The model under review builds one solid part; all positions refer to its coordinate system, in mm. A direction names the side the tool comes from. Round coordinates to 2 decimals unless told otherwise and drop trailing zeros. Loops run counter-clockwise (first coordinate to the right, second up) from the corner with the lowest first, then second, coordinate; pieces in that order, holes last. Notation, with made-up numbers: (88.5, 84) -> (130.5, 84) arc R22 ccw to (130.5, 92) -> close; hole circle Ø10 at (19, 9.5). An arc over 180 degrees is marked (long way). Use a Markdown table: item, result. Add a question column.
1) Wall thickness on probe 1 along Z at (x, y) = (-42.5, -19.5); probe 2 along Z at (x, y) = (1.5, -31.5); probe 3 along Z at (x, y) = (-49.5, -9): over which ranges is each line inside the solid? List them lowest first.
2) For faces 1 (the cylindrical face through (74.51, -17.26, -110.81)), 2 (the flat face through (-23, -25, 85)), list the 3-axis set-ups (+Z, -Z, +X, -X, +Y, -Y) from which the entire face can be reached by the end or side of a thin tool; tool diameter is ignored.
3) Consider section A-A on y = -13.5. Give the boundary of the cut face in (x, z), plus the area to 3 significant figures.
4) Consider section B-B on x = -41. Give the boundary of the cut face in (y, z), plus the area to 3 significant figures.
5) Consider section C-C on z = 111. Give the boundary of the cut face in (x, y).
6) Insertion check: pin 1 (2 mm diameter, centred on y = -16.5, z = -29.5, fed in from -X); pin 2 (2 mm diameter, centred on x = -67.5, y = -4, fed in from +Z); pin 3 (18 mm diameter, centred on x = -30, z = 91, fed in from -Y); pin 4 (4 mm diameter, centred on y = -31, z = 99.5, fed in from -X). Each pin has a flat end and moves straight along its axis. Give the tip position at first contact, or say it passes through.
7) Consider section D-D on z = -86. Give the boundary of the cut face in (x, y), plus the area to 3 significant figures.
8) Mouldability with a two-part tool opening along Z and no side actions: class faces 3 (the flat face through (-21, 0, -21)), 4 (the cylindrical face through (-71.99, -17.26, -117.1)), 5 (the cylindrical face through (1.054, -17.255, -91.871)) as released by +Z, released by -Z, zero draft, split by the parting line, or undercut.
from build123d import *

# Parameters (mm, degrees)
F1_DEPTH = 25
F0_R     = 16
F2_DEPTH = 35


with BuildPart() as f1:
    # F0 (on Front) → F1 (new body)
    with BuildSketch(Plane.XZ):
        with BuildLine():
            ThreePointArc((-6.260685, 97.864598), (-57.477963, 119.073727), (-36.249162, 67.864601))
            ThreePointArc((-36.249162, 67.864601), (-15.043408, 76.65547), (-6.260685, 97.864598))
        make_face()
        with BuildLine():
            ThreePointArc((-20.260685, 97.864598), (-24.942904, 86.554965), (-36.249162, 81.864603))
            ThreePointArc((-36.249162, 81.864603), (-47.578467, 109.174232), (-20.260685, 97.864598))
        make_face(mode=Mode.SUBTRACT)
        with BuildLine():
            ThreePointArc((-36.249162, -62.135402), (-50.391298, -96.277537), (-16.249162, -82.135402))
            ThreePointArc((-16.249162, -82.135402), (-22.107026, -67.993266), (-36.249162, -62.135402))
        make_face()
        with BuildLine():
            ThreePointArc((-26.249162, -82.135402), (-43.32023, -89.206469), (-36.249162, -72.135402))
            ThreePointArc((-36.249162, -72.135402), (-29.178094, -75.064334), (-26.249162, -82.135402))
        make_face(mode=Mode.SUBTRACT)
    extrude(amount=F1_DEPTH)

    # F0 (on Front) → F2 (join)
    with BuildSketch(Plane.XZ):
        with BuildLine():
            ThreePointArc((-26.249162, -82.135402), (-29.178094, -75.064334), (-36.249162, -72.135402))
            ThreePointArc((-36.249162, -72.135402), (-43.32023, -89.206469), (-26.249162, -82.135402))
        make_face()
        with BuildLine():
            ThreePointArc((-36.249162, -62.135402), (-50.391298, -96.277537), (-16.249162, -82.135402))
            ThreePointArc((-16.249162, -82.135402), (-22.107026, -67.993266), (-36.249162, -62.135402))
        make_face()
        with BuildLine():
            ThreePointArc((-26.249162, -82.135402), (-43.32023, -89.206469), (-36.249162, -72.135402))
            ThreePointArc((-36.249162, -72.135402), (-29.178094, -75.064334), (-26.249162, -82.135402))
        make_face(mode=Mode.SUBTRACT)
        with BuildLine():
            ThreePointArc((-20.260685, 97.864598), (-47.578467, 109.174232), (-36.249162, 81.864603))
            ThreePointArc((-36.249162, 81.864603), (-24.942904, 86.554965), (-20.260685, 97.864598))
        make_face()
        with BuildLine():
            ThreePointArc((-6.260685, 97.864598), (-57.477963, 119.073727), (-36.249162, 67.864601))
            ThreePointArc((-36.249162, 67.864601), (-15.043408, 76.65547), (-6.260685, 97.864598))
        make_face()
        with BuildLine():
            ThreePointArc((-20.260685, 97.864598), (-24.942904, 86.554965), (-36.249162, 81.864603))
            ThreePointArc((-36.249162, 81.864603), (-47.578467, 109.174232), (-20.260685, 97.864598))
        make_face(mode=Mode.SUBTRACT)
        with BuildLine():
            Line((80.040823, -63.740012), (13.198313, 105.199956))
            ThreePointArc((13.198313, 105.199956), (-39.402834, 147.76577), (-86.249162, 98.938004))
            Line((-86.249162, 98.938004), (-86.249162, 96.791193))
            Line((-86.249162, 96.791193), (-86.249162, -82.135402))
            ThreePointArc((-86.249162, -82.135402), (-71.604501, -117.490741), (-36.249162, -132.135402))
            Line((-36.249162, -132.135402), (33.547709, -132.135402))
            ThreePointArc((33.547709, -132.135402), (74.898462, -110.244391), (80.040823, -63.740012))
        make_face()
        with BuildLine():
            ThreePointArc((-36.249162, -62.135402), (-22.107026, -67.993266), (-16.249162, -82.135402))
            ThreePointArc((-16.249162, -82.135402), (-50.391298, -96.277537), (-36.249162, -62.135402))
        make_face(mode=Mode.SUBTRACT)
        with Locations((13.750838, -82.135402)):
            Circle(F0_R, mode=Mode.SUBTRACT)
        with BuildLine():
            ThreePointArc((-6.260685, 97.864598), (-15.043408, 76.65547), (-36.249162, 67.864601))
            ThreePointArc((-36.249162, 67.864601), (-57.477963, 119.073727), (-6.260685, 97.864598))
        make_face(mode=Mode.SUBTRACT)
        with BuildLine():
            Line((-86.249162, 96.791193), (-86.249162, 98.938004))
            ThreePointArc((-86.249162, 98.938004), (-86.260685, 97.864598), (-86.249162, 96.791193))
        make_face()
    extrude(amount=F2_DEPTH)


solid = f1.part
Result set:
| question | item | result |
|---|---|---|
| 1 | probe 1 | -131.74 to -89.94, -74.33 to 83.13, 112.6 to 147.47 |
| 1 | probe 2 | -132.14 to -92.43, -71.84 to 130.64 |
| 1 | probe 3 | -130.35 to 88.88, 106.85 to 146.08 |
| 2 | face 1 | +X, +Y, -Y |
| 2 | face 2 | -Y |
| 3 | outline | (-86.25, -82.14) arc R50 ccw to (-36.25, -132.14) -> (33.55, -132.14) arc R50 ccw to (80.04, -63.74) -> (13.2, 105.2) arc R50 ccw to (-86.25, 98.94) arc R50 ccw to (-86.25, 96.79) -> close; hole circle Ø20 at (-36.25, -82.14); hole (-36.25, 81.86) arc R16 ccw to (-20.26, 97.86) arc R16 ccw (long way) to start; hole circle Ø32 at (13.75, -82.14) |
| 3 | area | 34,200 mm2 |
| 4 | outline | (-35, -131.91) -> (0, -131.91) -> (0, -90.93) -> (-25, -90.93) -> (-25, -101.56) -> (-35, -101.56) -> close; (-35, -62.71) -> (-25, -62.71) -> (-25, -73.34) -> (0, -73.34) -> (0, 82.58) -> (-25, 82.58) -> (-25, 68.24) -> (-35, 68.24) -> close; (-35, 127.49) -> (-25, 127.49) -> (-25, 113.15) -> (0, 113.15) -> (0, 147.64) -> (-35, 147.64) -> close |
| 4 | area | 7,600 mm2 |
| 5 | outline | (-84.5, -35) -> (-63.23, -35) -> (-63.23, -25) -> (-45.4, -25) -> (-45.4, 0) -> (-84.5, 0) -> close; (-27.12, -25) -> (-9.29, -25) -> (-9.29, -35) -> (11.98, -35) -> (11.98, 0) -> (-27.12, 0) -> close |
| 6 | pin 1 | x = -86.25 |
| 6 | pin 2 | z = 137.68 |
| 6 | pin 3 | y = -25 |
| 6 | pin 4 | x = -86.26 |
| 7 | outline | (-86.1, -35) -> (-55.87, -35) -> (-55.87, -25) -> (-45.47, -25) -> (-45.47, 0) -> (-86.1, 0) -> close; (-27.03, -25) -> (-16.63, -25) -> (-16.63, -35) -> (-1.78, -35) -> (-1.78, 0) -> (-27.03, 0) -> close; (29.28, -35) -> (83.4, -35) -> (83.4, 0) -> (29.28, 0) -> close |
| 7 | area | 3,990 mm2 |
| 8 | face 3 | zero draft |
| 8 | face 4 | released by -Z |
| 8 | face 5 | undercut |
